from build123d import *

# Parameters (mm, degrees)
BOSS_EXTRUDE1_DEPTH = 37.465


with BuildPart() as part:
    # Sketch1 → Boss-Extrude1 (new, symmetric)
    with BuildSketch(Plane(origin=(0, 0, 0), x_dir=(0, 0, -1), z_dir=(1, 0, 0))):
        Polygon((7.332348419, 0), (3.666174209, 6.35), (-3.666174209, 6.35), (-7.332348419, 0), (-3.666174209, -6.35), (3.666174209, -6.35), align=None)
    extrude(amount=BOSS_EXTRUDE1_DEPTH, both=True)

    # Sketch2 → Cut-Revolve1 (revolve, cut)
    with BuildSketch(Plane(origin=(0, 0, 0), x_dir=(1, 0, 0), z_dir=(0, 1, 0))):
        Polygon((34.925, -5.8547), (35.9156, -5.8547), (35.9156, -6.35), (37.465, -6.35), (37.465, -8.89), (34.925, -8.89), align=None)
    cut_revolve1 = revolve(axis=Axis((0, 0, 0), (1, 0, 0)), mode=Mode.SUBTRACT)

    # Mirror1: Cut-Revolve1 across plane
    add(cut_revolve1.mirror(Plane(origin=(0, 0, 0), x_dir=(0, 0, 1), z_dir=(1, 0, 0))), mode=Mode.SUBTRACT)


solid = part.part
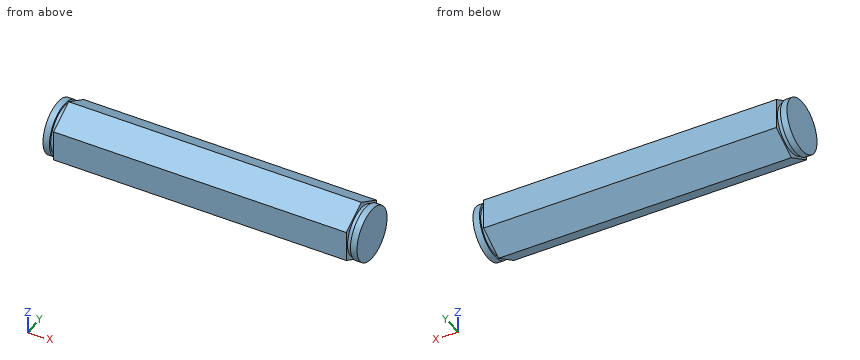
Here's how the part is built. I have some questions about the finished solid (model axes, mm). Coordinates: 2 decimals unless noted, no trailing zeros. Order: outer loops, then holes, each group sorted by start corner. A loop starts at its lowest first (then second) coordinate and runs counter-clockwise, first axis right, second up.
Item 1: For P1, Ø3, axis at x = -1.5, y = 2, coming from the +Z side; P2, Ø6, axis at x = 14, y = -1.5, coming from the +Z side; P3, Ø1.5, axis at x = -25, y = 5, coming from the -Z side, each with a flat end and sliding along its axis, tell me the tip position at first contact or that it passes through.
Result sheet:
P1: stops at z = 7.04
P2: stops at z = 7.33
P3: stops at z = -4.88
Item 2: If we section it at A-A on y = -2: List the corners of the cut face in (x, z) for me (1 decimal), plus the area to 3 significant figures.
Result sheet:
outline: (-37.5, -6) - (-35.9, -6) - (-35.9, -5.5) - (-34.9, -5.5) - (-34.9, -6.2) - (34.9, -6.2) - (34.9, -5.5) - (35.9, -5.5) - (35.9, -6) - (37.5, -6) - (37.5, 6) - (35.9, 6) - (35.9, 5.5) - (34.9, 5.5) - (34.9, 6.2) - (-34.9, 6.2) - (-34.9, 5.5) - (-35.9, 5.5) - (-35.9, 6) - (-37.5, 6) - close
area: 922 mm2
Item 3: I need wall thicknesses on line 1 (X direction, y = 0.5, z = -6.5) (3 decimals); line 2 (Y direction, x = -16, z = -4.5); line 3 (Z direction, x = 20, y = 5). Which ranges of each line are inside material? Lowest first, please.
Result sheet:
line 1: x = -34.925 to 34.925
line 2: y = -4.91 to 4.91
line 3: z = -4.45 to 4.45
Item 4: If we section it at B-B on x = -25: List the corners of the cut face in (y, z) for me, plus the area to 3 significant figures.
Result sheet:
outline: (-6.35, -3.67) - (0, -7.33) - (6.35, -3.67) - (6.35, 3.67) - (0, 7.33) - (-6.35, 3.67) - close
area: 140 mm2
Item 5: If we section it at C-C on y = 2.5: List the corners of the cut face in (x, z) for me (3 decimals), plus the area to 3 significant figures.
Result sheet:
outline: (-37.465, -5.837) - (-35.916, -5.837) - (-35.916, -5.294) - (-34.925, -5.294) - (-34.925, -5.889) - (34.925, -5.889) - (34.925, -5.294) - (35.916, -5.294) - (35.916, -5.837) - (37.465, -5.837) - (37.465, 5.837) - (35.916, 5.837) - (35.916, 5.294) - (34.925, 5.294) - (34.925, 5.889) - (-34.925, 5.889) - (-34.925, 5.294) - (-35.916, 5.294) - (-35.916, 5.837) - (-37.465, 5.837) - close
area: 880 mm2
